Work out the finished part from the listing and answer in its coordinate system (mm). A direction names the side the tool comes from. Give positions to 0.01 mm unless a question says otherwise; leave off trailing zeros. Write each loop counter-clockwise with the first axis right and the second up, starting at its lowest first coordinate (ties: lowest second). Pieces come first, ordered by that corner, then holes. Notation, with made-up numbers: (36.5, -14.75) -> (66.5, -14.75) arc R14 cw to (66.5, -5.75) -> close; hole circle Ø4 at (35, 27.25). An arc over 180 degrees is marked (long way). Use a Markdown table: item, result. Add a question column.
Q1. Each of these flat-tipped pins is pushed along its axis until it touches: pin 1 Ø5.5 at (x, y) = (-9, 35) entering from +Z; pin 2 Ø3 at (x, y) = (-5, 31) entering from -Z; pin 3 Ø5 at (x, y) = (-1, 20) entering from +Z; pin 4 Ø2 at (x, y) = (-27.5, 66.5) entering from -Z. Where does it stop, or does it pass through?
Q2. Section C-C, the plane y = 49 is taken. Give the vertices of the cut face in (x, z), plus the area to 3 significant figures.
Q3. For faces 5 (the face through (-39.05, 4.93, -8.67)), 6 (the face through (-26, 48, 0)), 7 (the face through (0, 19, -2.2)), determine the directions among +Z, -Z, +X, -X, +Y, -Y from which every point of the face is accessible in a straight line to the end or side of a thin tool.
Q4. For a pull along Z with two mould halves and no side action, classify faces 1 (the face through (-0.36, 40.25, -21.85)), 2 (the face through (0, 47, 10)), 3 (the face through (0, 57, 12)), 4 (the face through (-0.364, 40.101, 21.925)) as pulls with the +Z half, pulls with the -Z half, needs draft (parallel to the pull), parting line crosses it, or undercut.
Q5. Section A-A, the plane z = 0 is taken. State how many separate pieces and enclosed holes the cut face has, plus the area to 3 significant figures.
Q6. Consider line 1 (X direction, y = 66, z = 8.5); line 2 (Y direction, x = 11.5, z = -12); line 3 (Y direction, x = 0, z = -24). Determine where each line is inside the solid, lowest interval first.
Q7. Section B-B, the plane y = 63 is taken. Give the vertices of the cut face in (x, z), plus the area to 3 significant figures.
from build123d import *

# Parameters (mm, degrees)
SKETCH1_R               = 45
SKETCH1_R_2             = 40
BOSS_EXTRUDE1_DEPTH     = 10
BOSS_EXTRUDE2_START     = -15
SKETCH2_R               = 45
BOSS_EXTRUDE2_DEPTH     = 15
CHAMFER1_SIZE           = 10
CUT_EXTRUDE1_REACH      = 71.842
CUT_EXTRUDE1_END_RADIUS = 45
SKETCH4_R               = 2
SKETCH9_R               = 6
BOSS_EXTRUDE4_DEPTH     = 5
BOSS_EXTRUDE5_DEPTH     = 42
CUT_EXTRUDE2_REACH      = 87.434
BOSS_EXTRUDE6_DEPTH     = 5
SKETCH14_W              = 3
SKETCH14_H              = 20
BOSS_EXTRUDE7_DEPTH     = 42
FILLET1_START           = -27
FILLET1_DEPTH           = 54
FILLET2_START           = -27
FILLET2_DEPTH           = 54


with BuildPart() as part:
    # Sketch1 → Boss-Extrude1 (new body)
    with BuildSketch(Plane(origin=(0, 0, 0), x_dir=(1, 0, 0), z_dir=(0, 1, 0))):
        with Locations(Location((0, 0, 0), (0, 0, 270))):
            Circle(SKETCH1_R)
        with Locations(Location((0, 0, 0), (0, 0, 270))):
            Circle(SKETCH1_R_2, mode=Mode.SUBTRACT)
    extrude(amount=BOSS_EXTRUDE1_DEPTH)

    # Sketch2 → Boss-Extrude2 (add)
    with BuildSketch(Plane(origin=(0, 25, 0), x_dir=(1, 0, 0), z_dir=(0, 1, 0)).offset(BOSS_EXTRUDE2_START)):
        with Locations(Location((0, 0, 0), (0, 0, 270))):
            Circle(SKETCH2_R)
        with BuildLine():
            Line((-2.323790008, 2.2), (2.323790008, 2.2))
            ThreePointArc((2.323790008, 2.2), (0, -3.2), (-2.323790008, 2.2))
        make_face(mode=Mode.SUBTRACT)
    extrude(amount=BOSS_EXTRUDE2_DEPTH)

    # Chamfer1
    chamfer1_edges = [part.edges().sort_by_distance(p)[0] for p in [
        (0, 25, -45),
    ]]
    chamfer(chamfer1_edges, length=CHAMFER1_SIZE)

    # Cut-Extrude1: up to this cylinder (the profile starts inside it)
    cut_extrude1_end = Plane(origin=(0, 12.354135, 0), z_dir=(0, -1, 0)) * Cylinder(CUT_EXTRUDE1_END_RADIUS, 234.684, mode=Mode.PRIVATE)
    # Sketch4 → Cut-Extrude1 (cut, up to the surface)
    with BuildSketch(Plane.XY.offset(-2.2), mode=Mode.PRIVATE) as cut_extrude1_sk1:
        with Locations((0, 12.354134675)):
            Circle(SKETCH4_R)
    cut_extrude1_tool1 = extrude(cut_extrude1_sk1.sketch, amount=-CUT_EXTRUDE1_REACH, mode=Mode.PRIVATE) & cut_extrude1_end
    add(cut_extrude1_tool1.solids().sort_by_distance((0, 12.354135, -2.2))[0], mode=Mode.SUBTRACT)

    # Sketch9 → Boss-Extrude4 (add)
    with BuildSketch(Plane(origin=(21, 0, 0), x_dir=(0, 0, -1), z_dir=(1, 0, 0))):
        with BuildLine():
            Line((20, 25), (-20, 25))
            Line((-20, 25), (-10.246950766, 79))
            ThreePointArc((-10.246950766, 79), (0, 82), (10.246950766, 79))
            Line((10.246950766, 79), (20, 25))
        make_face()
        with Locations((0, 63)):
            Circle(SKETCH9_R, mode=Mode.SUBTRACT)
    boss_extrude4 = extrude(amount=BOSS_EXTRUDE4_DEPTH)

    # Mirror2: Boss-Extrude4 across plane
    add(boss_extrude4.mirror(Plane(origin=(0, 0, 0), x_dir=(0, 0, 1), z_dir=(1, 0, 0))))

    # Sketch10 → Boss-Extrude5 (add)
    with BuildSketch(Plane.ZY.offset(-21)):
        Polygon((-10, 57), (-14.220415269, 57), (-17.832655726, 37), (-10, 37), (-10, 52), align=None)
        Polygon((10, 52), (10, 57), (14.220415269, 57), (17.832655726, 37), (10, 37), align=None)
    extrude(amount=BOSS_EXTRUDE5_DEPTH)

    # Sketch11 → Cut-Extrude2 (cut, up to next)
    with BuildSketch(Plane(origin=(0, 25, 0), x_dir=(1, 0, 0), z_dir=(0, 1, 0)), mode=Mode.PRIVATE) as cut_extrude2_sk1:
        Polygon((-21, -17.832655726), (-21, -20), (21, -20), (21, -15), (-21, -15), align=None)
    cut_extrude2_tool1 = extrude(cut_extrude2_sk1.sketch, amount=-CUT_EXTRUDE2_REACH, mode=Mode.PRIVATE) & part.part
    add(cut_extrude2_tool1.solids().sort_by_distance((0, 25, 17.5))[0], mode=Mode.SUBTRACT)

    # Sketch13 → Boss-Extrude6 (add)
    with BuildSketch(Plane.ZY.offset(26)):
        Polygon((20, 25), (16.387759543, 45), (20, 45), (23, 45), (23, 25), align=None)
        Polygon((-23, 25), (-20, 25), (-16.387759543, 45), (-20, 45), (-23, 45), align=None)
    boss_extrude6 = extrude(amount=-BOSS_EXTRUDE6_DEPTH)

    # Mirror3: Boss-Extrude6 across plane
    add(boss_extrude6.mirror(Plane(origin=(0, 0, 0), x_dir=(0, 0, 1), z_dir=(1, 0, 0))))

    # Sketch14 → Boss-Extrude7 (add)
    with BuildSketch(Plane(origin=(-21, 0, 0), x_dir=(0, 0, -1), z_dir=(1, 0, 0))):
        with Locations((-21.5, 35)):
            Rectangle(SKETCH14_W, SKETCH14_H)
    boss_extrude7 = extrude(amount=BOSS_EXTRUDE7_DEPTH)

    # Mirror4: Boss-Extrude7 across plane
    add(boss_extrude7.mirror(Plane.XY))

    # Fillet1: read off the stored shape, not the designer's step
    # Fillet1 outline → Fillet1 (cut)
    with BuildSketch(Plane.YZ.offset(FILLET1_START)):
        with BuildLine():
            Line((45, 23), (35.59132925, 23))
            ThreePointArc((35.59132925, 23), (41.341216404, 21.181613393), (45, 16.387759543))
            Line((45, 16.387759543), (45, 23))
        make_face()
    extrude(amount=FILLET1_DEPTH, mode=Mode.SUBTRACT)

    # Fillet2: read off the stored shape, not the designer's step
    # Fillet2 outline → Fillet2 (cut)
    with BuildSketch(Plane.YZ.offset(FILLET2_START)):
        with BuildLine():
            Line((35.59132925, -23), (45, -23))
            Line((45, -23), (45, -16.387759543))
            ThreePointArc((45, -16.387759543), (41.341216404, -21.181613393), (35.59132925, -23))
        make_face()
    extrude(amount=FILLET2_DEPTH, mode=Mode.SUBTRACT)


solid = part.part
Result set:
| question | item | result |
|---|---|---|
| 1 | pin 1 | stops at z = 23 |
| 1 | pin 2 | stops at z = -23 |
| 1 | pin 3 | stops at z = 42.49 |
| 1 | pin 4 | passes through |
| 2 | outline | (-26, -15.67) -> (26, -15.67) -> (26, 15.67) -> (-26, 15.67) -> close; hole (-21, -10) -> (21, -10) -> (21, 10) -> (-21, 10) -> close |
| 2 | area | 789 mm2 |
| 3 | face 5 | -Y |
| 3 | face 6 | +Z, -Z, -X, +Y |
| 3 | face 7 | +Y, -Y |
| 4 | face 1 | pulls with the -Z half |
| 4 | face 2 | undercut |
| 4 | face 3 | needs draft |
| 4 | face 4 | pulls with the +Z half |
| 5 | separate pieces | 4 |
| 5 | enclosed holes | 0 |
| 5 | area | 1,700 mm2 |
| 6 | line 1 | x = -26 to -21, 21 to 26 |
| 6 | line 2 | y = 10 to 25, 37 to 57 |
| 6 | line 3 | y = 10 to 10.35, 14.35 to 25 |
| 7 | outline | (-26, -13.14) -> (-21, -13.14) -> (-21, -6) -> (-26, -6) -> close; (-26, 6) -> (-21, 6) -> (-21, 13.14) -> (-26, 13.14) -> close; (21, -13.14) -> (26, -13.14) -> (26, -6) -> (21, -6) -> close; (21, 6) -> (26, 6) -> (26, 13.14) -> (21, 13.14) -> close |
| 7 | area | 143 mm2 |
